Work out the finished part from the listing and answer in its coordinate system (mm). Coordinates: 2 decimals unless noted, no trailing zeros. Write each loop counter-clockwise with the first axis right and the second up, starting at its lowest first coordinate (ties: lowest second). Pieces come first, ordered by that corner, then holes. Notation, with made-up numbers: M 25,-28.5 L 38,-28.5 A22 cw 38,-22.5 Z; hole C -23.5,57 d5. An arc over 180 degrees is marked long. Answer as CSV lines item,"result". Start each with the question number.
(1) A cutting plane is placed at B-B on y = -0.75. Give the vertices of the cut face in (x, z).
(2) A cutting plane is placed at A-A on z = -8.25. Give the vertices of the cut face in (x, y), then the cut area to 3 significant figures.
(3) Flat-ended cylindrical pins translate along their axes: P1, Ø5, axis at x = 5.03, z = -7.94, coming from the -Y side; P2, Ø3, axis at x = -2.5, z = -17.5, coming from the +Y side; P3, Ø1, axis at y = -1, z = -18.5, coming from the +X side. Find the tip coordinate at first contact, or state that the pin passes through.
(4) A cutting plane is placed at C-C on x = -3.75. Give the vertices of the cut face in (y, z), then the cut area to 3 significant figures.
(5) A cutting plane is placed at D-D on z = -5.75. Give the vertices of the cut face in (x, y), then the cut area to 3 significant figures.
(6) Find the intervals of material crossed by L1, parallel to Y at x = 6, z = -16.75; L2, parallel to X at y = -1, z = -16.25; L3, parallel to X at y = -0.95, z = -8, in increasing order. Write a range as [from, to].
from build123d import *

# Parameters (mm, degrees)
F0_W     = 17.78
F0_H     = 22.86
F0_R     = 1.905
F1_DEPTH = 0.254
F2_R     = 1.397
F3_DEPTH = 3.81
F5_R     = 1.397
F6_DEPTH = 3.81
F8_R     = 1.397
F9_DEPTH = 3.81
F10_D    = 2.54


with BuildPart() as f1:
    # F0 (on Front) → F1 (new body)
    with BuildSketch(Plane.XZ):
        with Locations((-0.045063, -11.43)):
            Rectangle(F0_W, F0_H)
        with Locations((-2.585063, -18.415)):
            Circle(F0_R, mode=Mode.SUBTRACT)
        with Locations((5.034937, -14.9225)):
            Circle(F0_R, mode=Mode.SUBTRACT)
        with Locations((-2.585063, -11.43)):
            Circle(F0_R, mode=Mode.SUBTRACT)
        with Locations((-2.585063, -4.445)):
            Circle(F0_R, mode=Mode.SUBTRACT)
        with Locations((5.034937, -7.9375)):
            Circle(F0_R, mode=Mode.SUBTRACT)
    extrude(amount=F1_DEPTH)

    # F2 (on Top) → F3 (join)
    with BuildSketch(Plane.XY):
        with Locations((10.236152, 0)):
            Circle(F2_R)
    extrude(amount=-F3_DEPTH)

    # F5 (on offset) → F6 (join)
    with BuildSketch(Plane.XY.offset(-7.62)):
        with Locations((10.236152, 0)):
            Circle(F5_R)
    extrude(amount=-F6_DEPTH)

    # F8 (on offset) → F9 (join)
    with BuildSketch(Plane.XY.offset(-15.24)):
        with Locations((10.236152, 0)):
            Circle(F8_R)
    extrude(amount=-F9_DEPTH)

    # F10 (through all)
    with Locations(Plane.XY):
        with Locations((10.236152, 0)):
            Hole(F10_D / 2)


solid = f1.part
Here are the results:
1,outline,"M 9.06,-19.05 L 9.21,-19.05 L 9.21,-15.24 L 9.06,-15.24 Z; M 9.06,-11.43 L 9.21,-11.43 L 9.21,-7.62 L 9.06,-7.62 Z; M 9.06,-3.81 L 9.21,-3.81 L 9.21,0 L 9.06,0 Z; M 11.26,-19.05 L 11.41,-19.05 L 11.41,-15.24 L 11.26,-15.24 Z; M 11.26,-11.43 L 11.41,-11.43 L 11.41,-7.62 L 11.26,-7.62 Z; M 11.26,-3.81 L 11.41,-3.81 L 11.41,0 L 11.26,0 Z"
2,outline,"M -8.94,-0.25 L 3.16,-0.25 L 3.16,0 L -8.94,0 Z; M 6.91,-0.25 L 8.84,-0.25 L 8.84,-0.13 A1.4 ccw long 8.84,0 L 6.91,0 Z; hole C 10.24,0 d2.54"
2,area,"4.63 mm^2"
3,P1,"stops at y = -0.25"
3,P2,"stops at y = 0"
3,P3,"stops at x = 11.54"
4,outline,"M -0.25,-22.86 L 0,-22.86 L 0,-19.92 L -0.25,-19.92 Z; M -0.25,-16.91 L 0,-16.91 L 0,-12.94 L -0.25,-12.94 Z; M -0.25,-9.92 L 0,-9.92 L 0,-5.95 L -0.25,-5.95 Z; M -0.25,-2.94 L 0,-2.94 L 0,0 L -0.25,0 Z"
4,area,"3.51 mm^2"
5,outline,"M -8.94,-0.25 L -3.97,-0.25 L -3.97,0 L -8.94,0 Z; M -1.2,-0.25 L 8.84,-0.25 L 8.84,0 L -1.2,0 Z"
5,area,"3.81 mm^2"
6,L1,"y = [-0.25, 0]"
6,L2,"x = [9.26, 9.45], [11.02, 11.21]"
6,L3,"x = [9.21, 9.39], [11.08, 11.26]"
